from build123d import *

# Parameters (mm, degrees)
BOSS_EXTRUDE1_DEPTH                     = 4
CUT_EXTRUDE1_DEPTH                      = 3.5
BOSS_EXTRUDE2_DEPTH                     = 1
CBORE_FOR_M5_HEX_HEAD_BOLT1_D           = 4.5
CBORE_FOR_M5_HEX_HEAD_BOLT1_CBORE_D     = 8
CBORE_FOR_M5_HEX_HEAD_BOLT1_CBORE_DEPTH = 1.5


with BuildPart() as part:
    # Sketch1 → Boss-Extrude1 (new body)
    with BuildSketch(Plane.XY):
        with BuildLine():
            Line((-16, -9), (-16, 9))
            ThreePointArc((-16, 9), (0, 25), (16, 9))
            Line((16, 9), (16, -9))
            ThreePointArc((16, -9), (0, -25), (-16, -9))
        make_face()
    extrude(amount=BOSS_EXTRUDE1_DEPTH)

    # Sketch2 → Cut-Extrude1 (cut)
    with BuildSketch(Plane.XY.offset(4)):
        with BuildLine():
            Line((-5, -9), (-5, 9))
            ThreePointArc((-5, 9), (0, 14), (5, 9))
            Line((5, 9), (5, -9))
            ThreePointArc((5, -9), (0, -14), (-5, -9))
        make_face()
    extrude(amount=-CUT_EXTRUDE1_DEPTH, mode=Mode.SUBTRACT)

    # Sketch3 → Boss-Extrude2 (add)
    with BuildSketch(Plane.XY.offset(4)):
        with BuildLine():
            Line((16, -9), (16, 9))
            ThreePointArc((16, 9), (0, 25), (-16, 9))
            Line((-16, 9), (-16, -9))
            ThreePointArc((-16, -9), (0, -25), (16, -9))
        make_face()
        with BuildLine():
            Line((-15, 9), (-15, -9))
            ThreePointArc((-15, -9), (0, -24), (15, -9))
            Line((15, -9), (15, 9))
            ThreePointArc((15, 9), (0, 24), (-15, 9))
        make_face(mode=Mode.SUBTRACT)
    extrude(amount=BOSS_EXTRUDE2_DEPTH)

    # CBORE for M5 Hex Head Bolt1 (through all)
    with Locations(Plane.XY.offset(4)):
        with Locations((0, 17.9), (11, 0), (-11, 0), (0, -17.9)):
            CounterBoreHole(CBORE_FOR_M5_HEX_HEAD_BOLT1_D / 2, CBORE_FOR_M5_HEX_HEAD_BOLT1_CBORE_D / 2, CBORE_FOR_M5_HEX_HEAD_BOLT1_CBORE_DEPTH)


solid = part.part
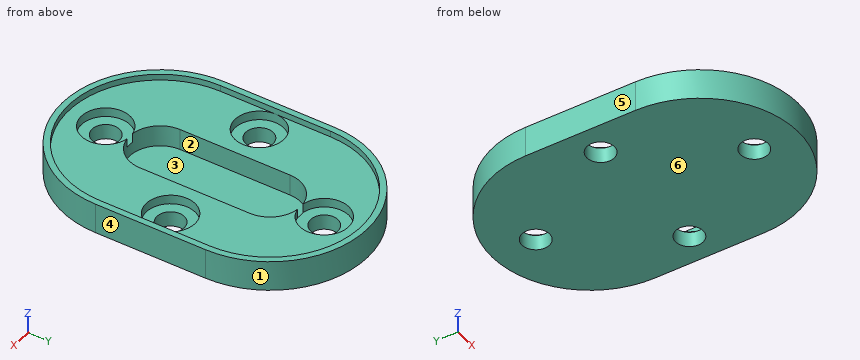
The listing builds one solid part. Answer for the finished solid, in the listing's coordinates (mm). Face numbers are marked on the shaded views. A direction names the side the tool comes from. Give positions to 0.01 mm unless a question says otherwise; leave off trailing zeros. Loops run counter-clockwise (first coordinate to the right, second up) from the corner with the lowest first, then second, coordinate; pieces in that order, holes last. Notation, with made-up numbers: (3, 47.25) - (50, 47.25) arc R12 cw to (50, 64.25) - close; hole circle Ø9 at (27.25, 60.25). An arc over 180 degrees is marked (long way). Answer as a JSON object with one key per item and string values.
1. Flat-ended cylindrical pins translate along their axes: pin 1 Ø8.5 at (x, y) = (-1.5, 19) entering from +Z; pin 2 Ø4 at (x, y) = (0, 17.9) entering from -Z; pin 3 Ø3 at (y, z) = (10.5, 3) entering from -X; pin 4 Ø6 at (x, y) = (-11, 0) entering from +Z. Find the tip coordinate at first contact, or state that the pin passes through.
Determined:
{"pin 1": "z = 4", "pin 2": "through", "pin 3": "x = -16", "pin 4": "z = 2.5"}
2. A cutting plane is placed at C-C (z = 3). Write down the section's boundary in (x, y), then the cut area to 3 significant figures.
Determined:
{"outline": "(-16, -9) arc R16 ccw to (16, -9) - (16, 9) arc R16 ccw to (-16, 9) - close; hole circle Ø8 at (-11, 0); hole (-5, -9) arc R5 ccw to (-0.66, -13.96) arc R4 ccw (long way) to (0.66, -13.96) arc R5 ccw to (5, -9) - (5, 9) arc R5 ccw to (0.66, 13.96) arc R4 ccw (long way) to (-0.66, 13.96) arc R5 ccw to (-5, 9) - close; hole circle Ø8 at (11, 0)", "area": "921 mm²"}
3. For the marked faces 1 and 2, determine the directions among +Z, -Z, +X, -X, +Y, -Y from which every point of the face is accessible in a straight line to the end or side of a thin tool.
Determined:
{"face 1": "+Z, -Z, +Y", "face 2": "+Z"}
4. A cutting plane is placed at A-A (x = 0). Write down the section's boundary in (y, z).
Determined:
{"outline": "(-25, 0) - (-20.15, 0) - (-20.15, 2.5) - (-21.9, 2.5) - (-21.9, 4) - (-24, 4) - (-24, 5) - (-25, 5) - close; (-15.65, 0) - (15.65, 0) - (15.65, 2.5) - (14, 2.5) - (14, 0.5) - (-14, 0.5) - (-14, 2.5) - (-15.65, 2.5) - close; (20.15, 0) - (25, 0) - (25, 5) - (24, 5) - (24, 4) - (21.9, 4) - (21.9, 2.5) - (20.15, 2.5) - close"}
5. For a pull along X with two mould halves and no side action, classify the marked faces 3, 4, 5 and 6 as pulls with the +X half, pulls with the -X half, needs draft (parallel to the pull), parting line crosses it, or undercut.
Determined:
{"face 3": "undercut", "face 4": "pulls with the +X half", "face 5": "pulls with the -X half", "face 6": "needs draft"}
6. Find the intervals of material crossed by L1, parallel to Y at x = 0, z = 1.7; L2, parallel to Y at x = 0, z = 3.2; L3, parallel to X at y = -7, z = 3.5, in increasing order. Write a range as [from, to].
Determined:
{"L1": "[-25, -20.15], [-15.65, -14], [14, 15.65], [20.15, 25]", "L2": "[-25, -21.9], [21.9, 25]", "L3": "[-16, -5], [5, 16]"}
7. A cutting plane is placed at B-B (y = 7). Write down the section's boundary in (x, z), then the cut area to 3 significant figures.
Determined:
{"outline": "(-16, 0) - (16, 0) - (16, 5) - (15, 5) - (15, 4) - (5, 4) - (5, 0.5) - (-5, 0.5) - (-5, 4) - (-15, 4) - (-15, 5) - (-16, 5) - close", "area": "95.0 mm²"}
8. A cutting plane is placed at D-D (x = -11.5). Write down the section's boundary in (y, z), then the cut area to 3 significant figures.
Determined:
{"outline": "(-20.12, 0) - (-2.19, 0) - (-2.19, 2.5) - (-3.97, 2.5) - (-3.97, 4) - (-18.63, 4) - (-18.63, 5) - (-20.12, 5) - close; (2.19, 0) - (20.12, 0) - (20.12, 5) - (18.63, 5) - (18.63, 4) - (3.97, 4) - (3.97, 2.5) - (2.19, 2.5) - close", "area": "141 mm²"}
